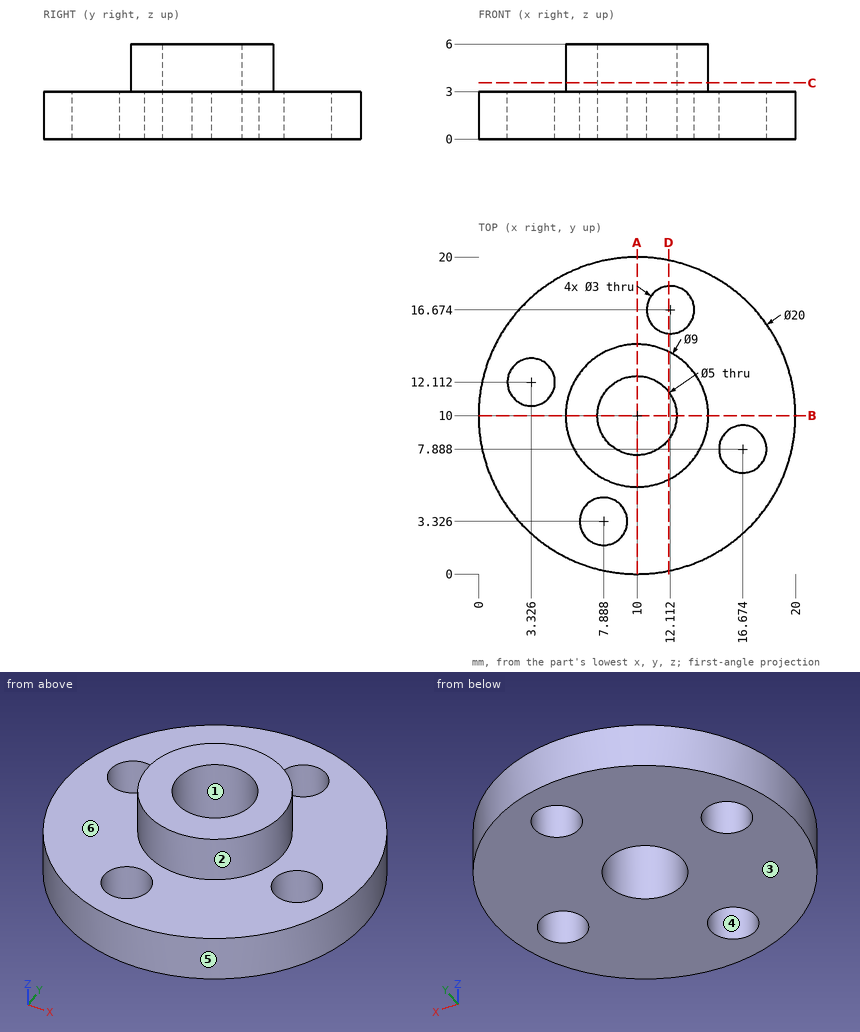
Geometry: see drawing. Coordinates: mm, zero at the bounding-box minimum. A direction names the side the tool comes from. Give positions to 0.01 mm unless a question says otherwise; leave off trailing zeros. Loops run counter-clockwise (first coordinate to the right, second up) from the corner with the lowest first, then second, coordinate; pieces in that order, holes last. Notation, with made-up numbers: (35, 59.5) -> (68, 59.5) arc R14 ccw to (68, 67.5) -> close; hole circle Ø1 at (14.5, -17.75). An arc over 180 degrees is marked (long way). Answer as a JSON object with one key per item and string values. Group by question number.
Item 1: Line query: probe 1 along Y at (x, z) = (9, 2.4); probe 2 along Y at (x, z) = (12, 1.85); probe 3 along Y at (x, z) = (10, 1.85). Output: solid intervals per line, ascending.
Item 2: Cut plane D-D, the plane x = 12. Return the cut outline in (y, z), and give its area (3 significant figures).
Item 3: Cut plane C-C, the plane z = 3.55. Return the cut outline in (x, y), and give its area (3 significant figures).
Item 4: Pull-direction query (Y, two-part tool) for the marked faces 1, 2, 3 and 4; classes: released by +Y, released by -Y, zero draft, split by the parting line, or undercut.
Item 5: Cut plane A-A, the plane x = 10. Return the cut outline in (y, z).
Item 6: Reachability of the marked faces 5 and 6 from +Z, -Z, +X, -X, +Y, -Y: full face, straight path, thin tool, end or side. Return the list, or none.
Item 7: Pin query (flat end, axial travel): P1, Ø2, axis at x = 12.5, z = 2, coming from the +Y side; P2, Ø2.5, axis at x = 12.11, y = 16.67, coming from the +Z side; P3, Ø1, axis at y = 5, z = 1, coming from the -X side; P4, Ø2, axis at x = 5, z = 2.5, coming from the +Y side (1 decimal). Return the tip coordinate at first contact, or that it passes through.
Checks:
{
 "1": {"probe 1": "y = 0.05 to 2.32, 4.33 to 7.71, 12.29 to 19.95", "probe 2": "y = 0.2 to 8.5, 11.5 to 15.18, 18.17 to 19.8", "probe 3": "y = 0 to 7.5, 12.5 to 20"},
 "2": {"outline": "(0.2, 0) -> (8.5, 0) -> (8.5, 6) -> (5.97, 6) -> (5.97, 3) -> (0.2, 3) -> close; (11.5, 0) -> (15.18, 0) -> (15.18, 3) -> (14.03, 3) -> (14.03, 6) -> (11.5, 6) -> close; (18.17, 0) -> (19.8, 0) -> (19.8, 3) -> (18.17, 3) -> close", "area": "56.0 mm²"},
 "3": {"outline": "circle Ø9 at (10, 10); hole circle Ø5 at (10, 10)", "area": "44.0 mm²"},
 "4": {"face 1": "undercut", "face 2": "split by the parting line", "face 3": "zero draft", "face 4": "undercut"},
 "5": {"outline": "(0, 0) -> (7.5, 0) -> (7.5, 6) -> (5.5, 6) -> (5.5, 3) -> (0, 3) -> close; (12.5, 0) -> (20, 0) -> (20, 3) -> (14.5, 3) -> (14.5, 6) -> (12.5, 6) -> close"},
 "6": {"face 5": "+Z, -Z", "face 6": "+Z"},
 "7": {"P1": "stops at y = 19.89", "P2": "passes through", "P3": "stops at x = 1.07", "P4": "stops at y = 19.2"}
}
